```python
from build123d import *

# Parameters (mm, degrees)
BASE_SKETCH_R        = 25
BOARD_DEPTH          = 1.6
ALIGNMENT_SLOTS_D    = 2
EXTRUSION_BASE_W     = 3
EXTRUSION_BASE_H     = 5.75
LEDS_DEPTH           = 1.1
EXTRUSION_BASE_3_W   = 5.15
EXTRUSION_BASE_3_H   = 5.15
EXTRUSION_BASE_3_W_2 = 3.1
EXTRUSION_BASE_3_H_2 = 3.1
ICS_DEPTH            = 1
EXTRUSION_BASE_4_W   = 2.85
EXTRUSION_BASE_4_H   = 8.15
CONNECTOR_DEPTH      = 1.3
EXTRA_MASS_CUT_DEPTH = 36.391524409


with BuildPart() as part:
    # Base sketch → Board (new body)
    with BuildSketch(Plane.XY):
        Circle(BASE_SKETCH_R)
    extrude(amount=BOARD_DEPTH)

    # Alignment slots (through all)
    with Locations(Plane.XY.offset(1.6)):
        with Locations((0, 25), (21.650635095, -12.5), (-21.650635095, -12.5)):
            Hole(ALIGNMENT_SLOTS_D / 2)

    # Extrusion base → LEDs (add)
    with BuildSketch(Plane(origin=(0, 0, 0), x_dir=(-1, 0, 0), z_dir=(0, 0, -1))):
        Polygon((10.039823036, 17.112559808), (11.539823036, 14.514483597), (6.560176964, 11.639483597), (5.060176964, 14.237559808), align=None)
        with Locations((-8.3, 14.376021703)):
            Rectangle(EXTRUSION_BASE_W, EXTRUSION_BASE_H)
        Polygon((19.839823036, -0.138461894), (18.339823036, -2.736538106), (13.360176964, 0.138461894), (14.860176964, 2.736538106), align=None)
        with Locations((8.3, -14.376021703)):
            Rectangle(EXTRUSION_BASE_W, EXTRUSION_BASE_H)
        Polygon((-10.039823036, -17.112559808), (-11.539823036, -14.514483597), (-6.560176964, -11.639483597), (-5.060176964, -14.237559808), align=None)
        Polygon((-19.839823036, 0.138461894), (-18.339823036, 2.736538106), (-13.360176964, -0.138461894), (-14.860176964, -2.736538106), align=None)
    extrude(amount=LEDS_DEPTH)

    # Extrusion base_3 → ICs (add)
    with BuildSketch(Plane(origin=(0, 0, 0), x_dir=(-1, 0, 0), z_dir=(0, 0, -1))):
        with Locations((1.3, 3.5)):
            Rectangle(EXTRUSION_BASE_3_W, EXTRUSION_BASE_3_H)
        with Locations((2.5, -3.2)):
            Rectangle(EXTRUSION_BASE_3_W_2, EXTRUSION_BASE_3_H_2)
    extrude(amount=ICS_DEPTH)

    # Extrusion base_4 → Connector (add)
    with BuildSketch(Plane(origin=(0, 0, 0), x_dir=(-1, 0, 0), z_dir=(0, 0, -1))):
        with Locations((-8.92, 0)):
            Rectangle(EXTRUSION_BASE_4_W, EXTRUSION_BASE_4_H)
    extrude(amount=CONNECTOR_DEPTH)

    # Negative base → Extra mass cut (cut, through all)
    with BuildSketch(Plane(origin=(0, 0, 0), x_dir=(-1, 0, 0), z_dir=(0, 0, -1))):
        with BuildLine():
            ThreePointArc((-18.83047802, -12.315157227), (-11.25, -19.485571585), (-1.25, -22.465250945))
            Line((-1.25, -22.465250945), (-1.25, -19.889716774))
            Line((-1.25, -19.889716774), (-8.05, -15.963734943))
            Line((-8.05, -15.963734943), (-10.039823036, -17.112559808))
            Line((-10.039823036, -17.112559808), (-11.539823036, -14.514483597))
            Line((-11.539823036, -14.514483597), (-11.05, -14.231684136))
            Line((-11.05, -14.231684136), (-16.6, -11.027390142))
            Line((-16.6, -11.027390142), (-18.83047802, -12.315157227))
        make_face()
        Polygon((-1.25, -17.002965428), (-1.25, -2.165063509), (-14.1, -9.584014469), (-8.55, -12.788308463), (-6.560176964, -11.639483597), (-5.060176964, -14.237559808), (-5.55, -14.52035927), align=None)
        Polygon((9.8, -12.066620626), (14.1, -9.584014469), (4.05, -3.781644263), (4.05, -4.75), (1.25, -4.75), (1.25, -17.002965428), (6.8, -13.798671434), (6.8, -11.501021703), (9.8, -11.501021703), align=None)
        with BuildLine():
            ThreePointArc((1.25, -22.465250945), (11.25, -19.485571585), (18.83047802, -12.315157227))
            Line((18.83047802, -12.315157227), (16.6, -11.027390142))
            Line((16.6, -11.027390142), (9.8, -14.953371972))
            Line((9.8, -14.953371972), (9.8, -17.251021703))
            Line((9.8, -17.251021703), (6.8, -17.251021703))
            Line((6.8, -17.251021703), (6.8, -16.68542278))
            Line((6.8, -16.68542278), (1.25, -19.889716774))
            Line((1.25, -19.889716774), (1.25, -22.465250945))
        make_face()
        Polygon((15.35, 2.453738644), (15.35, 7.418950959), (2.5, 0), (15.35, -7.418950959), (15.35, -1.010362971), (13.360176964, 0.138461894), (14.860176964, 2.736538106), align=None)
        with BuildLine():
            ThreePointArc((22.5, 0), (21.886762614, 5.217242784), (20.08047802, 10.150093718))
            Line((20.08047802, 10.150093718), (17.85, 8.862326632))
            Line((17.85, 8.862326632), (17.85, 1.010362971))
            Line((17.85, 1.010362971), (19.839823036, -0.138461894))
            Line((19.839823036, -0.138461894), (18.339823036, -2.736538106))
            Line((18.339823036, -2.736538106), (17.85, -2.453738644))
            Line((17.85, -2.453738644), (17.85, -8.862326632))
            Line((17.85, -8.862326632), (20.08047802, -10.150093718))
            ThreePointArc((20.08047802, -10.150093718), (21.886762614, -5.217242784), (22.5, 0))
        make_face()
        Polygon((3.875, 3.680607966), (14.1, 9.584014469), (8.55, 12.788308463), (6.560176964, 11.639483597), (5.060176964, 14.237559808), (5.55, 14.52035927), (1.25, 17.002965428), (1.25, 6.075), (3.875, 6.075), align=None)
        with BuildLine():
            Line((11.05, 14.231684136), (16.6, 11.027390142))
            Line((16.6, 11.027390142), (18.83047802, 12.315157227))
            ThreePointArc((18.83047802, 12.315157227), (11.25, 19.485571585), (1.25, 22.465250945))
            Line((1.25, 22.465250945), (1.25, 19.889716774))
            Line((1.25, 19.889716774), (8.05, 15.963734943))
            Line((8.05, 15.963734943), (10.039823036, 17.112559808))
            Line((10.039823036, 17.112559808), (11.539823036, 14.514483597))
            Line((11.539823036, 14.514483597), (11.05, 14.231684136))
        make_face()
        Polygon((-1.275, 6.075), (-1.25, 6.075), (-1.25, 17.002965428), (-6.8, 13.798671434), (-6.8, 11.501021703), (-9.8, 11.501021703), (-9.8, 12.066620626), (-14.1, 9.584014469), (-1.275, 2.179497266), align=None)
        with BuildLine():
            Line((-1.25, 19.889716774), (-1.25, 22.465250945))
            ThreePointArc((-1.25, 22.465250945), (-11.25, 19.485571585), (-18.83047802, 12.315157227))
            Line((-18.83047802, 12.315157227), (-16.6, 11.027390142))
            Line((-16.6, 11.027390142), (-9.8, 14.953371972))
            Line((-9.8, 14.953371972), (-9.8, 17.251021703))
            Line((-9.8, 17.251021703), (-6.8, 17.251021703))
            Line((-6.8, 17.251021703), (-6.8, 16.68542278))
            Line((-6.8, 16.68542278), (-1.25, 19.889716774))
        make_face()
        with BuildLine():
            Line((-9.558107041, 4.075), (-20.08047802, 10.150093718))
            ThreePointArc((-20.08047802, 10.150093718), (-21.733331092, 5.823428515), (-22.465250945, 1.25))
            Line((-22.465250945, 1.25), (-19.198076211, 1.25))
            Line((-19.198076211, 1.25), (-18.339823036, 2.736538106))
            Line((-18.339823036, 2.736538106), (-15.765063509, 1.25))
            Line((-15.765063509, 1.25), (-10.345, 1.25))
            Line((-10.345, 1.25), (-10.345, 4.075))
            Line((-10.345, 4.075), (-9.558107041, 4.075))
        make_face()
        with BuildLine():
            Line((-17.434936491, -1.25), (-22.465250945, -1.25))
            ThreePointArc((-22.465250945, -1.25), (-21.733331092, -5.823428515), (-20.08047802, -10.150093718))
            Line((-20.08047802, -10.150093718), (-9.558107041, -4.075))
            Line((-9.558107041, -4.075), (-10.345, -4.075))
            Line((-10.345, -4.075), (-10.345, -1.25))
            Line((-10.345, -1.25), (-14.001923789, -1.25))
            Line((-14.001923789, -1.25), (-14.860176964, -2.736538106))
            Line((-14.860176964, -2.736538106), (-17.434936491, -1.25))
        make_face()
        Polygon((-7.495, -2.883864595), (-2.5, 0), (-7.495, 2.883864595), align=None)
    extrude(amount=-EXTRA_MASS_CUT_DEPTH, mode=Mode.SUBTRACT)


solid = part.part
```
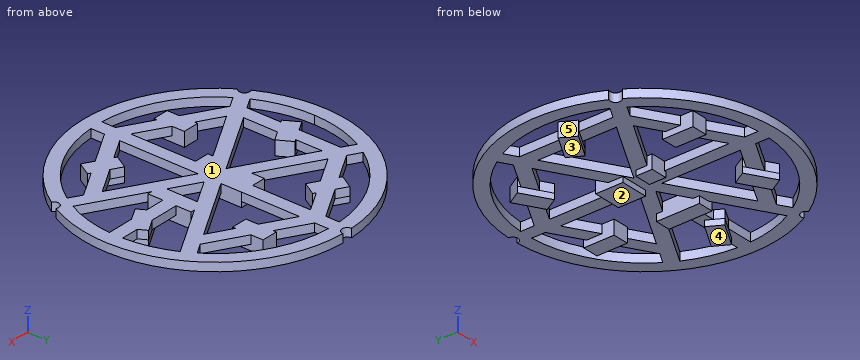
Part model, mm, in its own coordinate system. Face numbers are marked on the shaded views. A direction names the side the tool comes from. Coordinates: 2 decimals unless noted, no trailing zeros. Write each loop counter-clockwise with the first axis right and the second up, starting at its lowest first coordinate (ties: lowest second). Pieces come first, ordered by that corner, then holes.
Item 1: Slice it at B-B (y = -18.5). Write the cut outline in (x, z).
Item 2: Mould opens along Y. For the marked faces 4 and 5 say: released by +Y, released by -Y, zero draft, split by the parting line, or undercut.
Item 3: Slice it at C-C (y = -6). Write the cut outline in (x, z).
Item 4: Slice it at A-A (x = 0). Write the cut outline in (y, z) (3 decimals), and give its area (4 significant figures).
Item 5: Probe line 1 (Y direction, x = -17.5, z = 0.6); line 2 (Y direction, x = -14.5, z = 0.95); line 3 (X direction, y = 9.5, z = 0.2). List the from-to ranges inside material, lowest first.
Item 6: Which spindle directions (+Z, -Z, +X, -X, +Y, -Y) get a long thin tool onto all of the face, cutting with end or side? Do the marked faces 1, 2 and 3. Say none if no direction does.
Item 7: Pin check, flat tips, straight feed: pin 1 (1.4 mm diameter, centred on x = -9, z = 0, fed in from +Y); pin 2 (0.8 mm diameter, centred on y = 4, z = 0, fed in from -X); pin 3 (8 mm diameter, centred on x = -9, y = -5.5, fed in from -Z). Stop position of each tip, or through.
Results found:
1. outline: (-16.82, 0) - (-12.81, 0) - (-12.81, 1.6) - (-16.82, 1.6) - close; (-3.66, 0) - (3.66, 0) - (3.66, 1.6) - (-3.66, 1.6) - close; (12.81, 0) - (16.82, 0) - (16.82, 1.6) - (12.81, 1.6) - close
2. face 4: zero draft
2. face 5: undercut
3. outline: (-24.27, 0) - (-21.69, 0) - (-21.69, 1.6) - (-24.27, 1.6) - close; (-17.85, 0) - (-15.35, 0) - (-15.35, 1.6) - (-17.85, 1.6) - close; (-12.89, 0) - (-7.89, 0) - (-7.89, 1.6) - (-12.89, 1.6) - close; (-1.25, 0) - (1.25, 0) - (1.25, 1.6) - (-1.25, 1.6) - close; (7.89, 0) - (12.89, 0) - (12.89, 1.6) - (7.89, 1.6) - close; (21.69, 0) - (24.27, 0) - (24.27, 1.6) - (21.69, 1.6) - close
4. outline: (-25, 0) - (0.925, 0) - (0.925, -1) - (6.075, -1) - (6.075, 0) - (24, 0) - (24, 1.6) - (-25, 1.6) - close
4. area: 83.55 mm2
5. line 1: y = -17.85 to -14.14, -11.55 to 11.55, 14.14 to 17.85
5. line 2: y = -20.37 to -17.2, -12.24 to -6.93, -0.52 to 2.11, 6.93 to 12.24, 17.2 to 20.37
5. line 3: x = -23.12 to -20.4, -18.95 to -13.95, -1.25 to 1.25, 13.95 to 18.95, 20.4 to 23.12
6. face 1: +Z, +X, -X, +Y, -Y
6. face 2: -Z, +Y, -Y
6. face 3: -Z, -X, +Y, -Y
7. pin 1: stops at y = 23.58
7. pin 2: stops at x = -24.74
7. pin 3: stops at z = 0
